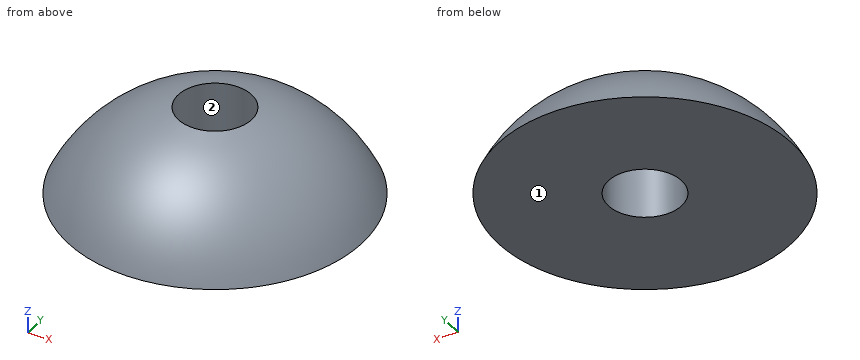
```python
from build123d import *

# Parameters (mm, degrees)
SKETCH6_R           = 22.5
SKETCH6_R_2         = 1
CUT_EXTRUDE8_DEPTH  = 20
SKETCH7_R           = 7.9
CUT_EXTRUDE9_DEPTH  = 20
SKETCH9_W           = 74.911016849
SKETCH9_H           = 74.606087337
CUT_EXTRUDE11_DEPTH = 50


with BuildPart() as part:
    # Sketch2 → Revolve1 (revolve)
    with BuildSketch(Plane.XY):
        with BuildLine():
            Line((0, 0), (70, 0))
            ThreePointArc((70, 0), (35, 35), (0, 0))
        make_face()
    revolve(axis=Axis((0, 0, 0), (1, 0, 0)))

    # Sketch6 → Cut-Extrude8 (cut)
    with BuildSketch(Plane.XY.offset(-5)):
        with Locations((35, -7)):
            Circle(SKETCH6_R)
        with Locations((17.5, -7)):
            Circle(SKETCH6_R_2, mode=Mode.SUBTRACT)
        with Locations((52.5, -7)):
            Circle(SKETCH6_R_2, mode=Mode.SUBTRACT)
    extrude(amount=CUT_EXTRUDE8_DEPTH, mode=Mode.SUBTRACT)

    # Sketch7 → Cut-Extrude9 (cut)
    with BuildSketch(Plane.XY.offset(35)):
        with Locations((35, 0)):
            Circle(SKETCH7_R)
    extrude(amount=-CUT_EXTRUDE9_DEPTH, mode=Mode.SUBTRACT)

    # Sketch9 → Cut-Extrude11 (cut)
    with BuildSketch(Plane.XY.offset(-35)):
        with Locations((35.457394269, -0.10164317)):
            Rectangle(SKETCH9_W, SKETCH9_H)
    extrude(amount=CUT_EXTRUDE11_DEPTH, mode=Mode.SUBTRACT)


solid = part.part
```
CAD build for the part. Positions are in the model's coordinates, mm. Face numbers are marked on the shaded views. Coordinates: 2 decimals unless noted, no trailing zeros. Write each loop counter-clockwise with the first axis right and the second up, starting at its lowest first coordinate (ties: lowest second). Pieces come first, ordered by that corner, then holes. Notation, with made-up numbers: (59.5, 76.5) -> (66.5, 76.5) arc R16 cw to (66.5, 89.5) -> close; hole circle Ø6 at (-22, 34). An arc over 180 degrees is marked (long way). Return JSON: item names as keys, results as strings. Group by question number.
Q1. Flat gauge pins, fed straight in: pin 1 (6 mm diameter, centred on y = -16, z = 23.5, fed in from +X); pin 2 (3 mm diameter, centred on y = 3.5, z = 23, fed in from -X); pin 3 (5 mm diameter, centred on x = 60, y = -4.5, fed in from +Z); pin 4 (9.5 mm diameter, centred on x = 35, y = 0, fed in from -Z). Where does each tip first touch, or does it go through?
Q2. Cut at D-D, the plane y = -9. Give the cut face in (x, z).
Q3. Pull direction X, two halves, no side cores. Call the marked faces 1 and 2: released by +X, released by -X, zero draft, split by the parting line, or undercut.
Q4. Cut at B-B, the plane x = 35. Give the cut face in (y, z), then the cut area to 3 significant figures.
Q5. Cut at C-C, the plane x = 17. Give the cut face in (y, z), then the cut area to 3 significant figures.
Q6. Cut at A-A, the plane y = 0. Give the cut face in (x, z), then the cut area to 3 significant figures.
Q7. Drill centre lines: line 1 (Y direction, x = 35, z = 28.5); line 2 (Y direction, x = 35, z = 26.5); line 3 (Z direction, x = 54, y = 25). Where is each one in solid material? Low to high.
Returned:
{
 "1": {"pin 1": "stops at x = 59.05", "pin 2": "stops at x = 7.59", "pin 3": "stops at z = 26.47", "pin 4": "passes through"},
 "2": {"outline": "(4.68, 15) -> (65.32, 15) arc R33.82 ccw to start"},
 "3": {"face 1": "zero draft", "face 2": "undercut"},
 "4": {"outline": "(-31.62, 15) -> (-7.9, 15) -> (-7.9, 34.1) arc R35 ccw to start; (7.9, 15) -> (31.62, 15) arc R35 ccw to (7.9, 34.1) -> close", "area": "596 mm2"},
 "5": {"outline": "(-26, 15) -> (26, 15) arc R30.02 ccw to start", "area": "554 mm2"},
 "6": {"outline": "(3.38, 15) -> (27.1, 15) -> (27.1, 34.1) arc R35 ccw to start; (42.9, 15) -> (66.62, 15) arc R35 ccw to (42.9, 34.1) -> close", "area": "596 mm2"},
 "7": {"line 1": "y = -20.32 to -7.9, 7.9 to 20.32", "line 2": "y = -22.86 to -7.9, 7.9 to 22.86", "line 3": "z = 15 to 15.46"}
}
